For this review, take the finished solid that the model builds, in its own axes (mm). Face numbers are marked on the shaded views. Round coordinates to 2 decimals unless told otherwise and drop trailing zeros. Loops run counter-clockwise (first coordinate to the right, second up) from the corner with the lowest first, then second, coordinate; pieces in that order, holes last. Notation, with made-up numbers: M 61.5,79 L 117.5,79 A34 cw 117.5,113 Z; hole C 54,1.25 d5. An arc over 180 degrees is marked long. One line per question, with ' | ' between items. Start each with the question number.
1) For pin 1 Ø1.5 at (x, y) = (0, 0) entering from +Z, flat-tipped, find the tip position at first contact; note if it passes through.
2) Mouldability with a two-part tool opening along Z and no side actions: class the marked faces 1, 2 and 3 as pulls with the +Z half, pulls with the -Z half, needs draft (parallel to the pull), parting line crosses it, or undercut.
3) For probe 1 along Z at (x, y) = (0, 2.8), list the stretches that pass through material, from the lowest coordinate up. Write a range as from..to.
4) We need section A-A (z = 3.5). Give the boundary of the cut face in (x, y), and give its area (3 significant figures).
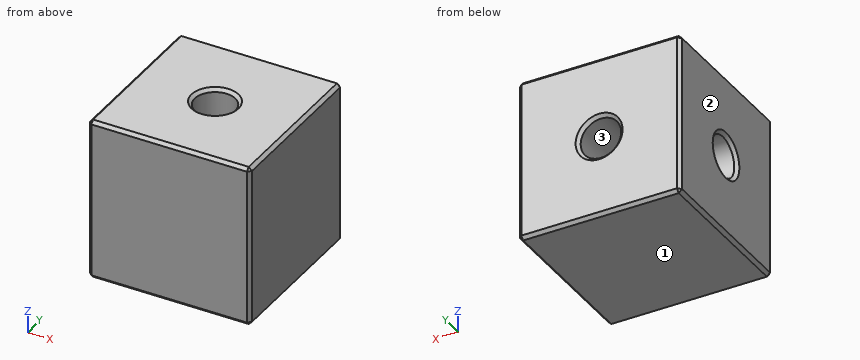
```python
from build123d import *
from OCP.BRepAlgoAPI import BRepAlgoAPI_Cut
from OCP.TopTools import TopTools_ListOfShape

# Parameters (mm, degrees)
SKETCH_1_W                 = 10
SKETCH_1_H                 = 10
EXTRUDE_1_DEPTH            = 5
HOLE_WIZARD_M3_1_D         = 2.5
HOLE_WIZARD_M3_1_DEPTH     = 4.999
HOLE_WIZARD_M3_2_OUTLINE_R = 1.25
HOLE_WIZARD_M3_2_DEPTH     = 5
HOLE_START                 = -5
HOLE_WIZARD_M3_3_OUTLINE_R = 1.25
HOLE_WIZARD_M3_3_DEPTH     = 5
CHAMFER_1_SIZE             = 0.2


with BuildPart() as part:
    # 草图1 → 凸台-拉伸1 (new, symmetric)
    with BuildSketch(Plane(origin=(0, 0, 0), x_dir=(1, 0, 0), z_dir=(0, 1, 0))):
        Rectangle(SKETCH_1_W, SKETCH_1_H)
    extrude(amount=EXTRUDE_1_DEPTH, both=True)

    # M3 螺纹孔1
    with Locations(Plane.XY.offset(5)):
        with Locations((0, 0)):
            Hole(HOLE_WIZARD_M3_1_D / 2, depth=HOLE_WIZARD_M3_1_DEPTH)


with BuildPart() as hole_wizard_m3_2_tool:
    # M3 螺纹孔2: read off the stored shape, not the designer's step
    # M3 螺纹孔2 outline → M3 螺纹孔2 (new body)
    with BuildSketch(Plane(origin=(0, 0, 0), x_dir=(1, 0, 0), z_dir=(0, 1, 0))):
        Circle(HOLE_WIZARD_M3_2_OUTLINE_R)
    extrude(amount=HOLE_WIZARD_M3_2_DEPTH)


with BuildPart() as part_1:
    add(part.part)

    # M3 螺纹孔2: cut by hole_wizard_m3_2_tool, with a tolerance
    hole_wizard_m3_2_stock = TopTools_ListOfShape()
    hole_wizard_m3_2_stock.Append(part_1.part.wrapped)
    hole_wizard_m3_2_tools = TopTools_ListOfShape()
    hole_wizard_m3_2_tools.Append(hole_wizard_m3_2_tool.part.wrapped)
    hole_wizard_m3_2_cut = BRepAlgoAPI_Cut()
    hole_wizard_m3_2_cut.SetArguments(hole_wizard_m3_2_stock)
    hole_wizard_m3_2_cut.SetTools(hole_wizard_m3_2_tools)
    hole_wizard_m3_2_cut.SetFuzzyValue(0.00001)
    hole_wizard_m3_2_cut.Build()
    add(Compound.cast(hole_wizard_m3_2_cut.Shape()).solids(), mode=Mode.REPLACE)

    # M3 螺纹孔3: read off the stored shape, not the designer's step
    # M3 螺纹孔3 outline → M3 螺纹孔3 (cut)
    with BuildSketch(Plane.YZ.offset(HOLE_START)):
        Circle(HOLE_WIZARD_M3_3_OUTLINE_R)
    extrude(amount=HOLE_WIZARD_M3_3_DEPTH, mode=Mode.SUBTRACT)

    # 草图7 → 切除-旋转1 (revolve, cut)
    with BuildSketch(Plane(origin=(0, 0, 0), x_dir=(1, 0, 0), z_dir=(0, 1, 0))):
        with BuildLine():
            Line((-1.25, 0), (1.25, 0))
            ThreePointArc((1.25, 0), (0, 1.25), (-1.25, 0))
        make_face()
    revolve(axis=Axis((0, 0, 0), (-1, 0, 0)), mode=Mode.SUBTRACT)

    # 倒角1
    chamfer_1_edges = [part_1.edges().sort_by_distance(p)[0] for p in [
        (-5, 5, 0),
        (1.25, 0, 5),
        (0, 5, 5),
        (-1.25, 5, 0),
        (-5, -1.25, 0),
        (5, 5, 0),
        (0, -5, 5),
        (-5, -5, 0),
        (0, -5, -5),
        (5, -5, 0),
        (5, 0, 5),
        (-5, 0, 5),
        (-5, 0, -5),
        (5, 0, -5),
        (0, 5, -5),
    ]]
    chamfer(chamfer_1_edges, length=CHAMFER_1_SIZE)


solid = part_1.part
```
Answers below:
1) pin 1: z = -1
2) face 1: pulls with the -Z half | face 2: needs draft | face 3: undercut
3) probe 1: -5..-1.25, 1.25..5
4) outline: M -5,-4.8 L -4.8,-5 L 4.8,-5 L 5,-4.8 L 5,4.8 L 4.8,5 L -4.8,5 L -5,4.8 Z; hole C 0,0 d2.5 | area: 95.0 mm^2
